```python
from build123d import *

# Parameters (mm, degrees)
F0_W     = 10
F0_H     = 10
F0_W_2   = 7.5
F0_H_2   = 7.5
F0_W_3   = 6.5
F0_H_3   = 6.5
F1_DEPTH = 20
F2_SIZE2 = 1
F2_SIZE  = 3
F3_SIZE2 = 1
F3_SIZE  = 3
F4_SIZE2 = 1
F4_SIZE  = 3
F5_SIZE2 = 1
F5_SIZE  = 3


with BuildPart() as f1:
    # F0 (on Top) → F1 (new body)
    with BuildSketch(Plane.XY):
        Rectangle(F0_W, F0_H)
        Rectangle(F0_W_2, F0_H_2, mode=Mode.SUBTRACT)
        Rectangle(F0_W_2, F0_H_2)
        Rectangle(F0_W_3, F0_H_3, mode=Mode.SUBTRACT)
    extrude(amount=F1_DEPTH)

    # F2
    f2_edges = [f1.edges().sort_by_distance(p)[0] for p in [
        (-3.25, 0, 20),
    ]]
    f2_side = f1.faces().sort_by_distance((-3.25, 0, 10))[0]
    chamfer(f2_edges, length=F2_SIZE, length2=F2_SIZE2, reference=f2_side)

    # F3
    f3_edges = [f1.edges().sort_by_distance(p)[0] for p in [
        (0, 3.25, 20),
    ]]
    f3_side = f1.faces().sort_by_distance((-0.040875, 3.25, 10.102662))[0]
    chamfer(f3_edges, length=F3_SIZE, length2=F3_SIZE2, reference=f3_side)

    # F4
    f4_edges = [f1.edges().sort_by_distance(p)[0] for p in [
        (3.25, 0, 20),
    ]]
    f4_side = f1.faces().sort_by_distance((3.25, 0.040875, 10.102662))[0]
    chamfer(f4_edges, length=F4_SIZE, length2=F4_SIZE2, reference=f4_side)

    # F5
    f5_edges = [f1.edges().sort_by_distance(p)[0] for p in [
        (0, -3.25, 20),
    ]]
    f5_side = f1.faces().sort_by_distance((0, -3.25, 10.203008))[0]
    chamfer(f5_edges, length=F5_SIZE, length2=F5_SIZE2, reference=f5_side)


solid = f1.part
```
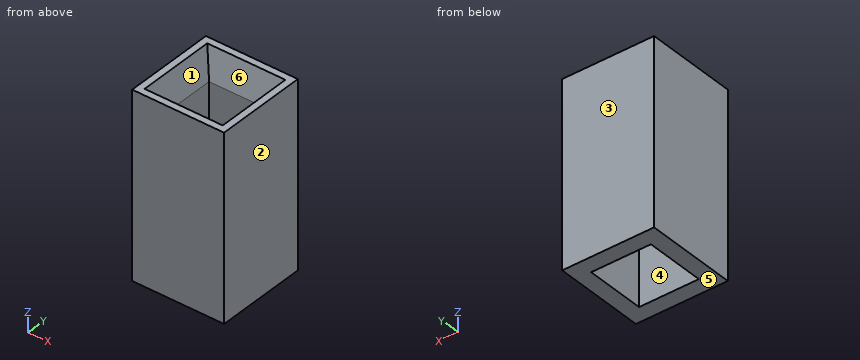
Can you work these out from the model? Positions are in its coordinate system, mm. Face numbers are marked on the shaded views. A direction names the side the tool comes from. Coordinates: 2 decimals unless noted, no trailing zeros. Loops run counter-clockwise (first coordinate to the right, second up) from the corner with the lowest first, then second, coordinate; pieces in that order, holes last.
1) Which directions (+Z, -Z, +X, -X, +Y, -Y) give clear straight access to the entire face, cutting with the end or side of a thin tool? Please do the marked faces 4, 5 and 6.
2) I need wall thicknesses on probe 1 along X at (y, z) = (-3, 2); probe 2 along Y at (x, z) = (3, 18). Which ranges of each line are inside material? Lowest first, please.
3) Imagine slicing it at D-D on y = 3.5. List the corners of the cut face in (x, z) for me.
4) Imagine slicing it at A-A on x = -2. List the corners of the cut face in (y, z) for me, plus the area to 3 significant figures.
5) Thinking about a two-plate mould opening in X: for the marked faces 1, 2 and 3, which applies, pulls with the +X half, pulls with the -X half, needs draft (parallel to the pull), parting line crosses it, or undercut?
6) Imagine slicing it at C-C on z = 15.5. List the corners of the cut face in (x, y) for me.
Completed:
1. face 4: +Z, -Z
1. face 5: -Z, +X, -X, +Y, -Y
1. face 6: +Z
2. probe 1: x = -5 to -3.25, 3.25 to 5
2. probe 2: y = -5 to -3.58, 3.58 to 5
3. outline: (-5, 0) - (5, 0) - (5, 20) - (4.25, 20) - (3.5, 17.75) - (-3.5, 17.75) - (-4.25, 20) - (-5, 20) - close
4. outline: (-5, 0) - (-3.25, 0) - (-3.25, 17) - (-4.25, 20) - (-5, 20) - close; (3.25, 0) - (5, 0) - (5, 20) - (4.25, 20) - (3.25, 17) - close
4. area: 67.0 mm2
5. face 1: undercut
5. face 2: pulls with the +X half
5. face 3: needs draft
6. outline: (-5, -5) - (5, -5) - (5, 5) - (-5, 5) - close; hole (-3.25, -3.25) - (3.25, -3.25) - (3.25, 3.25) - (-3.25, 3.25) - close
